Read the model definition and answer for the solid it produces. Units are mm, in the model's axes. Face numbers are marked on the shaded views. Give positions to 0.01 mm unless a question says otherwise; leave off trailing zeros. Order: outer loops, then holes, each group sorted by start corner. A loop starts at its lowest first (then second) coordinate and runs counter-clockwise, first axis right, second up.
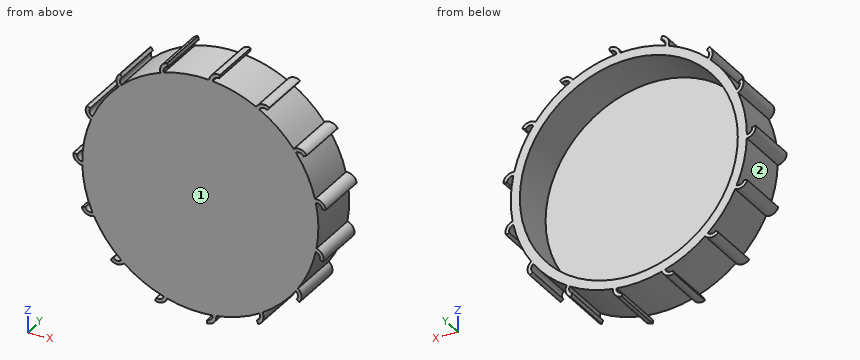
Autodesk Inventor part; units mm, degrees
ref_plane "YZ Plane" through (0, 0, 0) normal (1, 0, 0) x (0, 1, 0)
ref_plane "XZ Plane" through (0, 0, 0) normal (0, 1, 0) x (-1, 0, 0)
ref_plane "XY Plane" through (0, 0, 0) normal (0, 0, 1) x (1, 0, 0)
sketch "スケッチ1" plane through (0, 0, 0) normal (1, 0, 0) x (0, 1, 0)
  point P0 (0, 0)
sketch "スケッチ2" plane through (0, 0, 0) normal (0, 1, 0) x (-1, 0, 0)
  circle A0 centre (0, 0) radius 65
  dimension "d1" = 130
extrude "押し出し1" add sketch "スケッチ2" along normal blind 30
sketch "スケッチ3" plane through (0, 30, 0) normal (0, 1, 0) x (1, 0, 0)
  circle A0 centre (0, 0) radius 60
  dimension "d4" = 120
extrude "押し出し2" cut sketch "スケッチ3" against normal blind 25
sketch "スケッチ4" plane through (0, 0, 0) normal (0, -1, 0) x (1, 0, 0)
  circle A0 centre (0, 0) radius 65
  arc A1 (-64.9694, -1.9949) -> (-61.7673, -0.8673) centre (-64.9305, 3.005) ccw
  arc A2 (-69.9053, 3.5064) -> (-61.7673, -0.8673) centre (-64.9305, 3.005) ccw
  line L0 (-64.9305, 3.005) -> (-69.9053, 3.5064) construction
  line L1 (-64.9305, 3.005) -> (-61.7673, -0.8673) construction
  arc A3 (-67.9154, 3.3058) -> (-64.6802, 0.0154) centre (-64.9305, 3.005) ccw
  line L2 (-69.9053, 3.5064) -> (-67.9154, 3.3058)
  line L3 (-60.5392, -23.6644) -> (-65.2878, -25.2298) construction
  arc A4 (-63.3884, -24.6037) -> (-59.0946, -26.2937) centre (-60.5392, -23.6644) ccw
  arc A5 (-65.2878, -25.2298) -> (-56.0745, -25.9153) centre (-60.5392, -23.6644) ccw
  line L4 (-65.2878, -25.2298) -> (-63.3884, -24.6037)
  line L5 (-45.6801, -46.242) -> (-49.3815, -49.6035) construction
  arc A6 (-47.901, -48.2589) -> (-43.291, -48.0565) centre (-45.6801, -46.242) ccw
  arc A7 (-49.3815, -49.6035) -> (-40.6859, -46.4824) centre (-45.6801, -46.242) ccw
  line L6 (-49.3815, -49.6035) -> (-47.901, -48.2589)
  line L7 (-22.9225, -60.824) -> (-24.9367, -65.4004) construction
  arc A8 (-24.131, -63.5698) -> (-20.002, -61.5098) centre (-22.9225, -60.824) ccw
  arc A9 (-24.9367, -65.4004) -> (-18.2623, -59.0122) centre (-22.9225, -60.824) ccw
  line L8 (-24.9367, -65.4004) -> (-24.131, -63.5698)
  line L9 (3.7986, -64.8889) -> (3.8199, -69.8889) construction
  arc A10 (3.8114, -67.8889) -> (6.7456, -64.3275) centre (3.7986, -64.8889) ccw
  arc A11 (3.8199, -69.8889) -> (7.319, -61.3383) centre (3.7986, -64.8889) ccw
  line L10 (3.8199, -69.8889) -> (3.8114, -67.8889)
  line L11 (29.8629, -57.734) -> (31.916, -62.293) construction
  arc A12 (31.0948, -60.4694) -> (32.3267, -56.0225) centre (29.8629, -57.734) ccw
  arc A13 (31.916, -62.293) -> (31.6347, -53.0584) centre (29.8629, -57.734) ccw
  line L12 (31.916, -62.293) -> (31.0948, -60.4694)
  line L13 (50.7636, -40.5963) -> (54.4936, -43.926) construction
  arc A14 (53.0016, -42.5941) -> (52.3183, -38.0306) centre (50.7636, -40.5963) ccw
  arc A15 (54.4936, -43.926) -> (50.4806, -35.6043) centre (50.7636, -40.5963) ccw
  line L14 (54.4936, -43.926) -> (53.0016, -42.5941)
  line L15 (62.8868, -16.4391) -> (67.6487, -17.9639) construction
  arc A16 (65.7439, -17.354) -> (63.2636, -13.4629) centre (62.8868, -16.4391) ccw
  arc A17 (67.6487, -17.9639) -> (60.5979, -11.9938) centre (62.8868, -16.4391) ccw
  line L16 (67.6487, -17.9639) -> (65.7439, -17.354)
  line L17 (64.1364, 10.5605) -> (69.1067, 11.1044) construction
  arc A18 (67.1186, 10.8868) -> (63.27, 13.4327) centre (64.1364, 10.5605) ccw
  arc A19 (69.1067, 11.1044) -> (60.2372, 13.6905) centre (64.1364, 10.5605) ccw
  line L18 (69.1067, 11.1044) -> (67.1186, 10.8868)
  line L19 (54.2962, 35.7341) -> (58.6156, 38.2526) construction
  arc A20 (56.8878, 37.2452) -> (52.3365, 38.0056) centre (54.2962, 35.7341) ccw
  arc A21 (58.6156, 38.2526) -> (49.4611, 37.0076) centre (54.2962, 35.7341) ccw
  line L20 (58.6156, 38.2526) -> (56.8878, 37.2452)
  line L21 (35.0676, 54.729) -> (37.9893, 58.7866) construction
  arc A22 (36.8206, 57.1635) -> (32.3535, 56.007) centre (35.0676, 54.729) ccw
  arc A23 (37.9893, 58.7866) -> (30.1326, 53.9257) centre (35.0676, 54.729) ccw
  line L22 (37.9893, 58.7866) -> (36.8206, 57.1635)
  line L23 (9.7756, 64.2607) -> (10.7943, 69.1558) construction
  arc A24 (10.3868, 67.1978) -> (6.7763, 64.3243) centre (9.7756, 64.2607) ccw
  arc A25 (10.7943, 69.1558) -> (5.5939, 61.5196) centre (9.7756, 64.2607) ccw
  line L24 (10.7943, 69.1558) -> (10.3868, 67.1978)
  line L25 (-17.2067, 62.6812) -> (-18.2672, 67.5674) construction
  arc A26 (-17.843, 65.6129) -> (-19.9726, 61.5193) centre (-17.2067, 62.6812) ccw
  arc A27 (-18.2672, 67.5674) -> (-19.912, 58.4762) centre (-17.2067, 62.6812) ccw
  line L26 (-18.2672, 67.5674) -> (-17.843, 65.6129)
  line L27 (-41.2138, 50.2635) -> (-44.17, 54.296) construction
  arc A28 (-42.9876, 52.683) -> (-43.268, 48.0771) centre (-41.2138, 50.2635) ccw
  arc A29 (-44.17, 54.296) -> (-41.9749, 45.3218) centre (-41.2138, 50.2635) ccw
  line L28 (-44.17, 54.296) -> (-42.9876, 52.683)
  line L29 (-58.0947, 29.1548) -> (-62.4355, 31.6363) construction
  arc A30 (-60.6992, 30.6437) -> (-59.0821, 26.3219) centre (-58.0947, 29.1548) ccw
  arc A31 (-62.4355, 31.6363) -> (-56.78, 24.3308) centre (-58.0947, 29.1548) ccw
  line L30 (-62.4355, 31.6363) -> (-60.6992, 30.6437)
  point P0 (-21.9739, 61.1731)
  point P1 (-20.0806, 61.8205)
  point P2 (4.8072, 64.822)
  point P3 (6.8001, 64.6433)
  point P4 (30.7571, 57.2626)
  point P5 (32.505, 56.2888)
  point P6 (51.3888, 39.8019)
  point P7 (52.5895, 38.2014)
  point P8 (63.1349, 15.4592)
  point P9 (63.5808, 13.5086)
  point P10 (63.9644, -11.5566)
  point P11 (63.5784, -13.5199)
  point P12 (53.7339, -36.5742)
  point P13 (52.5827, -38.2107)
  point P14 (34.2123, -55.2677)
  point P15 (32.495, -56.2945)
  point P16 (8.7751, -64.405)
  point P17 (6.7886, -64.6445)
  point P18 (-18.1794, -62.406)
  point P19 (-20.0916, -61.8169)
  point P20 (-41.9905, -49.6165)
  point P21 (-43.4978, -48.3005)
  point P22 (-58.5411, -28.2478)
  point P23 (-59.3828, -26.4326)
  point P24 (-44.9555, 46.9468)
  point P25 (-43.4892, 48.3083)
  point P26 (-60.1639, 24.603)
  point P27 (-59.3781, 26.4432)
  point P28 (-64.9694, -1.9949)
  point P29 (-65, 0.0058)
  dimension "d8" = 5
  dimension "d9" = 135
  dimension "d10" = 3
  dimension "d13" = 360
sketch "スケッチ5" plane through (0, 0, 0) normal (0, -1, 0) x (1, 0, 0)
  circle A0 centre (0, 0) radius 65
  line L0 (-65, 0) -> (-64.9694, -1.9932)
sketch "スケッチ6" plane through (0, 0, 0) normal (0, -1, 0) x (1, 0, 0)
  point P0 (0, 0)
extrude "押し出し3" add sketch "スケッチ4" against normal blind 30 contours A0 A19 L18 A18 | A17 L16 A16 A0 | A0 A21 L20 A20 | A15 L14 A14 A0 | A0 A23 L22 A22 | A13 L12 A12 A0 | A0 A25 L24 A24 | A11 L10 A10 A0 | A0 A27 L26 A26 | A9 L8 A8 A0 | A0 A29 L28 A28 | A7 L6 A6 A0 | A0 A31 L30 A30 | A5 L4 A4 A0 | A0 A2 L2 A3
properties part number "wheel_rib_ant1"
1) Consider L1, parallel to Z at x = -47.5, y = 13.75; L2, parallel to X at y = 26.75, z = -26; L3, parallel to Z at x = 0, y = 10.75. Determine where each line is inside the solid, lowest interval first.
Final values:
L1: z = -50.9 to -48.63, -44.37 to -36.66, 36.66 to 44.37
L2: x = -64.96 to -62.42, -59.57 to -54.07, 54.07 to 59.57
L3: z = -65 to -60, 60 to 65
2) The part is cut by section A-A on x = 0. Determine the outline of the cut face in (y, z), and give its area (3 significant figures).
Final values:
outline: (0, -65) - (30, -65) - (30, -60) - (5, -60) - (5, 60) - (30, 60) - (30, 65) - (0, 65) - close
area: 900 mm2
3) For a pull along Z with two mould halves and no side action, classify the marked faces 1 and 2 as released by +Z, released by -Z, zero draft, split by the parting line, or undercut.
Final values:
face 1: zero draft
face 2: undercut
4) The part is cut by section B-B on z = 6.5. Determine the outline of the cut face in (x, y), and give its area (3 significant figures).
Final values:
outline: (-64.67, 0) - (64.67, 0) - (64.67, 30) - (59.65, 30) - (59.65, 5) - (-59.65, 5) - (-59.65, 30) - (-64.67, 30) - close
area: 898 mm2
5) Given pin 1 (3 mm diameter, centred on x = 15, y = 15.5, fed in from -Z); pin 2 (1 mm diameter, centred on y = 17, z = -28.5, fed in from +X); pin 3 (1 mm diameter, centred on y = 9.5, z = 42.5, fed in from -X), each flat-ended and moving along its own axis, determine where each tip first touches the part or whether it passes through.
Final values:
pin 1: stops at z = -63.58
pin 2: stops at x = 58.66
pin 3: stops at x = -49.61
